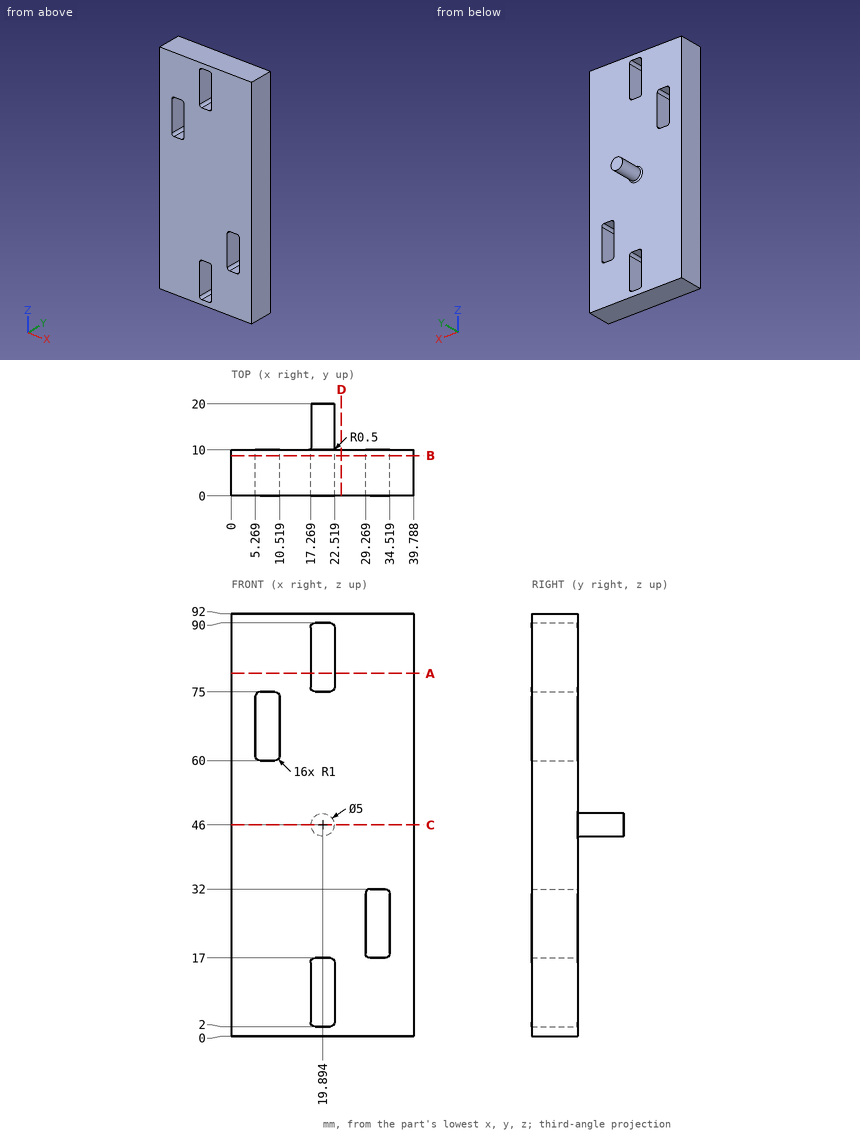
Here's the drawing with two shaded views (mm, measured from the low corner). I have some questions. Give positions to 0.01 mm unless a question says otherwise; leave off trailing zeros. Order: outer loops, then holes, each group sorted by start corner. A loop starts at its lowest first (then second) coordinate and runs counter-clockwise, first axis right, second up. Notation, with made-up numbers: M 75,-10.5 L 97,-10.5 A20 cw 97,-4.5 Z; hole C 50.5,38.5 d1. An arc over 180 degrees is marked long. One line per item, written item: value.
1) Please list where these lines run through material, in increasing order: line 1 along Z through (x, y) = (20.5, 6.5); line 2 along X through (y, z) = (7, 66); line 3 along X through (y, z) = (8.75, 22.5).
Answer sheet:
line 1: z = 0 to 2, 17 to 75, 90 to 92
line 2: x = 0 to 5.27, 10.52 to 39.79
line 3: x = 0 to 29.27, 34.52 to 39.79
2) I want a section at D-D, the plane x = 24. List the corners of the cut face in (y, z) for me, plus the area to 3 significant figures.
Answer sheet:
outline: M 0,0 L 10,0 L 10,92 L 0,92 Z
area: 920 mm^2
3) I want a section at B-B, the plane y = 8.75. Count the separate pieces of the cut face and the enclosed holes in it, plus the area to 3 significant figures.
Answer sheet:
separate pieces: 1
enclosed holes: 4
area: 3,350 mm^2
4) I want a section at C-C, the plane z = 46. List the corners of the cut face in (x, y) for me.
Answer sheet:
outline: M 0,0 L 39.79,0 L 39.79,10 L 22.89,10 A0.5 cw 22.39,10.5 L 22.39,20 L 17.39,20 L 17.39,10.5 A0.5 cw 16.89,10 L 0,10 Z
5) I want a section at A-A, the plane z = 79. List the corners of the cut face in (x, y) for me, plus the area to 3 significant figures.
Answer sheet:
outline: M 0,0 L 17.27,0 L 17.27,10 L 0,10 Z; M 22.52,0 L 39.79,0 L 39.79,10 L 22.52,10 Z
area: 345 mm^2
6) For P1, Ø4, axis at y = 13, z = 79.5, coming from the -X side; P2, Ø1, axis at x = 32.5, y = 5, coming from the -Z side; P3, Ø1.5, axis at x = 22, y = 14, coming from the +Z side, each with a flat end and sliding along its axis, tell me the tip position at first contact or that it passes through.
Answer sheet:
P1: passes through
P2: stops at z = 0
P3: stops at z = 48.1
